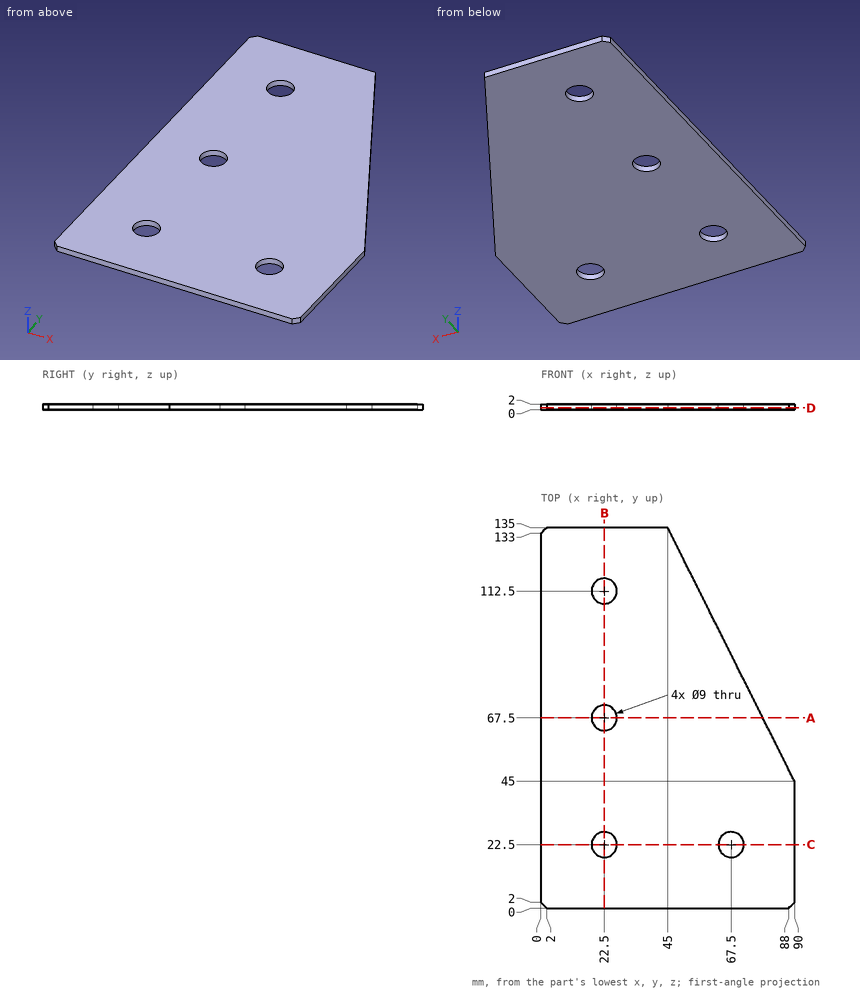
Here's the drawing with two shaded views (mm, measured from the low corner). I have some questions. Coordinates: 2 decimals unless noted, no trailing zeros. Loops run counter-clockwise (first coordinate to the right, second up) from the corner with the lowest first, then second, coordinate; pieces in that order, holes last. Notation, with made-up numbers: (7.25, 65) -> (32.25, 65) arc R15 ccw to (32.25, 71) -> close; hole circle Ø8 at (48, 75). An arc over 180 degrees is marked (long way). Put each result on its own line as item: value. Start each with the question number.
Q1. I want a section at A-A (y = 67.5). Write out the boundary of the cut face in (x, z), plus the area to 4 significant figures.
Q2. I want a section at B-B (x = 22.5). Write out the boundary of the cut face in (y, z).
Q3. I want a section at D-D (z = 0.6). Write out the boundary of the cut face in (x, y), plus the area to 3 significant figures.
Q4. If I drill on line 1 (Y direction, x = 22.5, z = 1.25); line 2 (X direction, y = 22.5, z = 1.65); line 3 (Y direction, x = 67.5, z = 0.45), over which ranges is the centre line in solid material (lowest first)? Write a range as [from, to].
Q5. I want a section at C-C (y = 22.5). Write out the boundary of the cut face in (x, z).
Taken from the geometry:
1. outline: (0, 0) -> (18, 0) -> (18, 2) -> (0, 2) -> close; (27, 0) -> (78.75, 0) -> (78.75, 2) -> (27, 2) -> close
1. area: 139.5 mm2
2. outline: (0, 0) -> (18, 0) -> (18, 2) -> (0, 2) -> close; (27, 0) -> (63, 0) -> (63, 2) -> (27, 2) -> close; (72, 0) -> (108, 0) -> (108, 2) -> (72, 2) -> close; (117, 0) -> (135, 0) -> (135, 2) -> (117, 2) -> close
3. outline: (0, 2) -> (2, 0) -> (88, 0) -> (90, 2) -> (90, 45) -> (45, 135) -> (2, 135) -> (0, 133) -> close; hole circle Ø9 at (22.5, 22.5); hole circle Ø9 at (22.5, 67.5); hole circle Ø9 at (22.5, 112.5); hole circle Ø9 at (67.5, 22.5)
3. area: 9,860 mm2
4. line 1: y = [0, 18], [27, 63], [72, 108], [117, 135]
4. line 2: x = [0, 18], [27, 63], [72, 90]
4. line 3: y = [0, 18], [27, 90]
5. outline: (0, 0) -> (18, 0) -> (18, 2) -> (0, 2) -> close; (27, 0) -> (63, 0) -> (63, 2) -> (27, 2) -> close; (72, 0) -> (90, 0) -> (90, 2) -> (72, 2) -> close
